Read the model definition and answer for the solid it produces. Units are mm, in the model's axes. A direction names the side the tool comes from. Coordinates: 2 decimals unless noted, no trailing zeros. Loops run counter-clockwise (first coordinate to the right, second up) from the corner with the lowest first, then second, coordinate; pieces in that order, holes last. Notation, with made-up numbers: M -36.75,2.25 L 0.25,2.25 A13 cw 0.25,17.25 Z; hole C -11,56.5 d8. An arc over 180 degrees is marked long. Put each result on its own line as item: value.
from build123d import *

# Parameters (mm, degrees)
BOSS_EXTRUDE1_DEPTH = 5
SKETCH2_R           = 2.1
CUT_EXTRUDE1_DEPTH  = 10
BOSS_EXTRUDE2_DEPTH = 5
BOSS_EXTRUDE3_DEPTH = 5
SKETCH5_R           = 2.1
CUT_EXTRUDE2_DEPTH  = 5
BOSS_EXTRUDE4_DEPTH = 5
SKETCH10_W          = 5.4
SKETCH10_H          = 15.4
SKETCH10_W_2        = 15.4
SKETCH10_H_2        = 5.4
SKETCH10_W_3        = 15
SKETCH10_H_3        = 5
CUT_EXTRUDE7_DEPTH  = 10
SKETCH11_W          = 15
SKETCH11_H          = 5
CUT_EXTRUDE8_DEPTH  = 10
SKETCH12_R          = 2.1
CUT_EXTRUDE9_DEPTH  = 10


with BuildPart() as part:
    # Sketch1 → Boss-Extrude1 (new body)
    with BuildSketch(Plane.XY):
        Polygon((-182, 200), (-182, 180), (-187, 180), (-187, 20), (-182, 20), (-182, 0), (0, 0), (0, 20), (5, 20), (5, 180), (0, 180), (0, 200), align=None)
    extrude(amount=BOSS_EXTRUDE1_DEPTH)

    # Sketch2 → Cut-Extrude1 (cut)
    with BuildSketch(Plane(origin=(0, 0, 0), x_dir=(-1, 0, 0), z_dir=(0, 0, -1))):
        with Locations((-2.5, 139.3)):
            Circle(SKETCH2_R)
        with Locations((-2.5, 37.9)):
            Circle(SKETCH2_R)
        with Locations(Location((184.5, 37.9, 0), (0, 0, 180))):
            Circle(SKETCH2_R)
        with Locations(Location((184.5, 139.3, 0), (0, 0, 180))):
            Circle(SKETCH2_R)
    extrude(amount=-CUT_EXTRUDE1_DEPTH, mode=Mode.SUBTRACT)

    # Sketch3 → Boss-Extrude2 (add)
    with BuildSketch(Plane(origin=(0, 0, 0), x_dir=(-1, 0, 0), z_dir=(0, 0, -1))):
        with BuildLine():
            Line((-5, 136.177501001), (-5, 142.422498999))
            ThreePointArc((-5, 142.422498999), (-6.5, 139.3), (-5, 136.177501001))
        make_face()
    boss_extrude2 = extrude(amount=-BOSS_EXTRUDE2_DEPTH)

    # Sketch4 → Boss-Extrude3 (add)
    with BuildSketch(Plane(origin=(0, 0, 0), x_dir=(-1, 0, 0), z_dir=(0, 0, -1))):
        with BuildLine():
            Line((-5, 34.777501001), (-5, 41.022498999))
            ThreePointArc((-5, 41.022498999), (-6.5, 37.9), (-5, 34.777501001))
        make_face()
    boss_extrude3 = extrude(amount=-BOSS_EXTRUDE3_DEPTH)

    # Mirror1: Boss-Extrude2, Boss-Extrude3 across plane
    add(boss_extrude2.mirror(Plane.ZY.offset(91)))
    add(boss_extrude3.mirror(Plane.ZY.offset(91)))

    # Sketch5 → Cut-Extrude2 (cut)
    with BuildSketch(Plane(origin=(0, 0, 0), x_dir=(-1, 0, 0), z_dir=(0, 0, -1))):
        with Locations((30, 2.5)):
            Circle(SKETCH5_R)
        with Locations((152, 2.5)):
            Circle(SKETCH5_R)
    extrude(amount=-CUT_EXTRUDE2_DEPTH, mode=Mode.SUBTRACT)

    # Sketch6 → Boss-Extrude4 (add)
    with BuildSketch(Plane(origin=(0, 0, 0), x_dir=(-1, 0, 0), z_dir=(0, 0, -1))):
        with BuildLine():
            Line((155.122498999, 0), (148.877501001, 0))
            ThreePointArc((148.877501001, 0), (152, -1.5), (155.122498999, 0))
        make_face()
        with BuildLine():
            Line((33.122498999, 0), (26.877501001, 0))
            ThreePointArc((26.877501001, 0), (30, -1.5), (33.122498999, 0))
        make_face()
    extrude(amount=-BOSS_EXTRUDE4_DEPTH)

    # Sketch10 → Cut-Extrude7 (cut)
    # profile 1 of 4: a face of its own
    with BuildSketch(Plane(origin=(0, 0, 0), x_dir=(-1, 0, 0), z_dir=(0, 0, -1))):
        with Locations((7.3, 91.747126042)):
            Rectangle(SKETCH10_W, SKETCH10_H)
    # profile 2 of 4: a face of its own
    with BuildSketch(Plane(origin=(0, 0, 0), x_dir=(-1, 0, 0), z_dir=(0, 0, -1))):
        with Locations((174.7, 91.747126042)):
            Rectangle(SKETCH10_W, SKETCH10_H)
    # profile 3 of 4: a face of its own
    with BuildSketch(Plane(origin=(0, 0, 0), x_dir=(-1, 0, 0), z_dir=(0, 0, -1))):
        with Locations((91, -4.005747915)):
            Rectangle(SKETCH10_W_2, SKETCH10_H_2)
        with Locations((91, -4.005747915)):
            Rectangle(SKETCH10_W_3, SKETCH10_H_3, mode=Mode.SUBTRACT)
    # profile 4 of 4: a face of its own
    with BuildSketch(Plane(origin=(0, 0, 0), x_dir=(-1, 0, 0), z_dir=(0, 0, -1))):
        with Locations((91, 187.5)):
            Rectangle(SKETCH10_W_2, SKETCH10_H_2)
        with Locations((91, 187.5)):
            Rectangle(SKETCH10_W_3, SKETCH10_H_3, mode=Mode.SUBTRACT)
    extrude(amount=-CUT_EXTRUDE7_DEPTH, mode=Mode.SUBTRACT)


with BuildPart() as cut_extrude7_piece_1:
    # of the separate pieces the step leaves, piece 1, a body of its own (cut_extrude7_pieces)
    add(part.part.solids().sort_by_distance((-182, 200, 0))[0])

    # Sketch12 → Cut-Extrude9 (cut)
    with BuildSketch(Plane.XY.offset(5)):
        with Locations((-108.5, 187.5)):
            Circle(SKETCH12_R)
        with Locations((-73.5, 187.5)):
            Circle(SKETCH12_R)
        with Locations((-73.5, -4.005747915)):
            Circle(SKETCH12_R)
        with Locations((-108.5, -4.005747915)):
            Circle(SKETCH12_R)
        with Locations((-174.7, 109.247126042)):
            Circle(SKETCH12_R)
        with Locations((-174.7, 74.247126042)):
            Circle(SKETCH12_R)
        with Locations((-7.3, 74.247126042)):
            Circle(SKETCH12_R)
        with Locations((-7.3, 109.247126042)):
            Circle(SKETCH12_R)
    extrude(amount=-CUT_EXTRUDE9_DEPTH, mode=Mode.SUBTRACT)


with BuildPart() as cut_extrude7_piece_2:
    # of the separate pieces the step leaves, piece 2, a body of its own (cut_extrude7_pieces)
    add(part.part.solids().sort_by_distance((-98.5, 185, 0))[0])

    # Sketch11 → Cut-Extrude8 (cut)
    with BuildSketch(Plane.XY.offset(5)):
        with Locations((-91, 12.499999997)):
            Rectangle(SKETCH11_W, SKETCH11_H)
        with Locations((-91, 187.5)):
            Rectangle(SKETCH11_W, SKETCH11_H)
    extrude(amount=-CUT_EXTRUDE8_DEPTH, mode=Mode.SUBTRACT)


solid = cut_extrude7_piece_1.part
1) Determine the mould class of faces 1 (the flat face through (-187, 161, 2)), 2 (the flat face through (2, 20, 2)), 3 (the flat face through (-83.3, 187, 2)) for opening direction X: released by +X, released by -X, zero draft, split by the parting line, or undercut.
Answer list:
face 1: released by -X
face 2: zero draft
face 3: undercut
2) Straight lines are drawn through the part: line 1 (Y direction, x = 2.5, z = 3.7); line 2 (Y direction, x = -7.5, z = 0.95); line 3 (X direction, y = 96, z = 2.8). For each, find the intervals that lie inside material, in ascending order. Write a range as [from, to].
Answer list:
line 1: y = [20, 35.8], [40, 137.2], [141.4, 180]
line 2: y = [0, 72.16], [76.34, 84.05], [99.45, 107.16], [111.34, 200]
line 3: x = [-187, -177.4], [-172, -10], [-4.6, 5]
3) Find section C-C, the plane y = 162.5. Write down the section's boundary in (x, z).
Answer list:
outline: M -187,0 L 5,0 L 5,5 L -187,5 Z
4) Given pin 1 Ø1.5 at (x, z) = (-184.5, 2.5) entering from -Y; pin 2 Ø6 at (x, y) = (-105.5, 112.5) entering from -Z; pin 3 Ø1.5 at (y, z) = (187, 1.5) entering from +X; pin 4 Ø2.5 at (x, y) = (-174.7, 109.25) entering from -Z, each flat-ended and moving along its own axis, determine where each tip first touches the part or whether it passes through.
Answer list:
pin 1: stops at y = 20
pin 2: stops at z = 0
pin 3: stops at x = 0
pin 4: passes through
5) Find section B-B, the plane z = 3.05. Count the separate pieces of the cut face and the enclosed holes in it, plus the area to 3 significant figures.
Answer list:
separate pieces: 1
enclosed holes: 15
area: 37,600 mm^2
6) Which of the six approach directions +Z, -Z, +X, -X, +Y, -Y give full straight-line access (tool end or side, diameter ignored) to faces 4 (the flat face through (-10, 92, 2)), 5 (the flat face through (5, 88, 2)), 6 (the flat face through (-184, 180, 2))?
Answer list:
face 4: +Z, -Z
face 5: +Z, -Z, +X
face 6: +Z, -Z, -X, +Y
7) Find section A-A, the plane y = 13. Write down the section's boundary in (x, z).
Answer list:
outline: M -182,0 L 0,0 L 0,5 L -182,5 Z
